```python
from build123d import *

# Parameters (mm, degrees)
F0_W      = 101.5
F0_H      = 85
F1_DEPTH  = 15.875
F3_DEPTH  = 25
F4_W      = 78.5
F4_H      = 15.875
F5_DEPTH  = 3.5
F6_W      = 78.5
F6_H      = 15.875
F7_DEPTH  = 3.5
F8_R      = 1.5
F8_W      = 66.5
F8_H      = 3
F8_W_2    = 72.5
F9_DEPTH  = 25
F10_W     = 72.5
F10_H     = 3
F10_W_2   = 66.5
F10_R     = 1.5
F11_DEPTH = 25
F12_R     = 2.5
F13_DEPTH = 5
F14_R     = 2.5
F15_DEPTH = 5
F16_R     = 2.5
F17_DEPTH = 5
F18_R     = 2.5
F19_DEPTH = 5
F20_R     = 1.5
F21_DEPTH = 10


with BuildPart() as f1:
    # F0 (on Front) → F1 (new body)
    with BuildSketch(Plane.XZ):
        Rectangle(F0_W, F0_H)
    extrude(amount=F1_DEPTH)

    # F2 (on face) → F3 (cut)
    with BuildSketch(Plane.XZ.offset(15.875)):
        with BuildLine():
            Line((-45.75, 31), (-45.75, -31))
            ThreePointArc((-45.75, -31), (-43.846194, -35.596194), (-39.25, -37.5))
            Line((-39.25, -37.5), (39.25, -37.5))
            ThreePointArc((39.25, -37.5), (43.846194, -35.596194), (45.75, -31))
            Line((45.75, -31), (45.75, 31))
            ThreePointArc((45.75, 31), (43.846194, 35.596194), (39.25, 37.5))
            Line((39.25, 37.5), (-39.25, 37.5))
            ThreePointArc((-39.25, 37.5), (-43.846194, 35.596194), (-45.75, 31))
        make_face()
    extrude(amount=-F3_DEPTH, mode=Mode.SUBTRACT)

    # F4 (on face) → F5 (cut)
    with BuildSketch(Plane.XY.offset(42.5)):
        with Locations((0, -7.9375)):
            Rectangle(F4_W, F4_H)
    extrude(amount=-F5_DEPTH, mode=Mode.SUBTRACT)

    # F6 (on face) → F7 (cut)
    with BuildSketch(Plane(origin=(0, 0, -42.5), x_dir=(1, 0, 0), z_dir=(0, 0, -1))):
        with Locations((0, 7.9375)):
            Rectangle(F6_W, F6_H)
    extrude(amount=-F7_DEPTH, mode=Mode.SUBTRACT)

    # F8 (on face) → F9 (cut)
    with BuildSketch(Plane.XY.offset(39)):
        with Locations((34.75, -4.5)):
            Circle(F8_R)
        with Locations((-3, -4.5)):
            Rectangle(F8_W, F8_H)
        with Locations((0, -10.5)):
            Rectangle(F8_W_2, F8_H)
    extrude(amount=-F9_DEPTH, mode=Mode.SUBTRACT)

    # F10 (on face) → F11 (cut)
    with BuildSketch(Plane(origin=(0, 0, -39), x_dir=(1, 0, 0), z_dir=(0, 0, -1))):
        with Locations((0, 10.5)):
            Rectangle(F10_W, F10_H)
        with Locations((3, 4.5)):
            Rectangle(F10_W_2, F10_H)
        with Locations((-34.75, 4.5)):
            Circle(F10_R)
    extrude(amount=-F11_DEPTH, mode=Mode.SUBTRACT)

    # F12 (on face) → F13 (cut)
    with BuildSketch(Plane(origin=(0, 0, -42.5), x_dir=(1, 0, 0), z_dir=(0, 0, -1))):
        with Locations((-45, 7.9375)):
            Circle(F12_R)
    extrude(amount=-F13_DEPTH, mode=Mode.SUBTRACT)

    # F14 (on face) → F15 (cut)
    with BuildSketch(Plane(origin=(0, 0, -42.5), x_dir=(1, 0, 0), z_dir=(0, 0, -1))):
        with Locations((45, 7.9375)):
            Circle(F14_R)
    extrude(amount=-F15_DEPTH, mode=Mode.SUBTRACT)

    # F16 (on face) → F17 (cut)
    with BuildSketch(Plane.XY.offset(42.5)):
        with Locations((-45, -7.9375)):
            Circle(F16_R)
    extrude(amount=-F17_DEPTH, mode=Mode.SUBTRACT)

    # F18 (on face) → F19 (cut)
    with BuildSketch(Plane.XY.offset(42.5)):
        with Locations((45, -7.9375)):
            Circle(F18_R)
    extrude(amount=-F19_DEPTH, mode=Mode.SUBTRACT)

    # F20 (on face) → F21 (cut)
    with BuildSketch(Plane.XZ.offset(15.875)):
        with Locations((-48.25, 25)):
            Circle(F20_R)
        with Locations((-48.25, 0)):
            Circle(F20_R)
        with Locations((-48.25, -25)):
            Circle(F20_R)
        with Locations((48.25, -25)):
            Circle(F20_R)
        with Locations((48.25, 0)):
            Circle(F20_R)
        with Locations((48.25, 25)):
            Circle(F20_R)
    extrude(amount=-F21_DEPTH, mode=Mode.SUBTRACT)


solid = f1.part
```
Check sheet for the modelled part. Datum: model origin and axes. Units: mm. A direction names the side the tool comes from. Round coordinates to 2 decimals unless told otherwise and drop trailing zeros. Write each loop counter-clockwise with the first axis right and the second up, starting at its lowest first coordinate (ties: lowest second). Pieces come first, ordered by that corner, then holes. Notation, with made-up numbers: (-16.75, 36.5) -> (17.25, 36.5) arc R15 ccw to (17.25, 50.5) -> close; hole circle Ø4 at (-1.75, -18.75). An arc over 180 degrees is marked (long way). One line per question, with ' | ' between items. Start each with the question number.
1. Set-up check for faces 4 (the face through (45, -8, 37.5)), 5 (the face through (39.25, -8, -41)), 6 (the face through (-43.795, -8.049, 35.646)), 7 (the face through (48, -5.875, -25)): record each of +Z, -Z, +X, -X, +Y, -Y from which the full face is reachable in a straight line by a thin tool's end or side.
2. Release check for a two-part mould opening along X. For faces 1 (the face through (-48, -8, 42.5)), 2 (the face through (47.309, -8.895, 40.035)), 3 (the face through (50.75, -8, -1)) record: +X half, -X half, draft (parallel to the pull), parting line (faces both ways), or undercut.
3. Sectioned sample at A-A, the plane x = -31.5. Record the cut outline in (y, z) (3 decimals).
4. Sectioned sample at C-C, the plane z = -25. Record the cut outline in (x, y) (3 decimals), then the cut area to 4 significant figures.
5. Depth check by flat-ended pin: pin 1 (2.5 mm diameter, centred on x = -48.25, z = 25, fed in from -Y) (3 decimals); pin 2 (1.5 mm diameter, centred on x = -16.5, y = -8.5, fed in from -Z); pin 3 (2.5 mm diameter, centred on x = -45, y = -7.5, fed in from -Z); pin 4 (8 mm diameter, centred on x = 39, z = 31, fed in from -Y). Enter the tip coordinate at first touch or a pass-through.
6. Scan lines: line 1 along Z through (x, y) = (-48.25, -12.5); line 2 along X through (y, z) = (-14.25, 4); line 3 along Z through (x, y) = (-13.5, -14.5). Record each from-to range of solid material in increasing order. Write a range as from..to.
7. Sectioned sample at B-B, the plane y = -14.75. Record the cut outline in (x, z).
8. Sectioned sample at D-D, the plane z = 17. Record the cut outline in (x, y) (3 decimals), then the cut area to 3 significant figures.
Taken from the geometry:
1) face 4: +Z | face 5: -Z, +Y, -Y | face 6: +Y, -Y | face 7: -Y
2) face 1: draft | face 2: undercut | face 3: +X half
3) outline: (-15.875, -39) -> (-12, -39) -> (-12, -37.5) -> (-15.875, -37.5) -> close; (-15.875, 37.5) -> (-12, 37.5) -> (-12, 39) -> (-15.875, 39) -> close; (-9, -39) -> (0, -39) -> (0, -37.5) -> (-9, -37.5) -> close; (-9, 37.5) -> (-6, 37.5) -> (-6, 39) -> (-9, 39) -> close; (-3, 37.5) -> (0, 37.5) -> (0, 39) -> (-3, 39) -> close
4) outline: (-50.75, -15.875) -> (-49.75, -15.875) -> (-49.75, -5.875) -> (-46.75, -5.875) -> (-46.75, -15.875) -> (-45.75, -15.875) -> (-45.75, 0) -> (-50.75, 0) -> close; (45.75, -15.875) -> (46.75, -15.875) -> (46.75, -5.875) -> (49.75, -5.875) -> (49.75, -15.875) -> (50.75, -15.875) -> (50.75, 0) -> (45.75, 0) -> close | area: 98.75 mm^2
5) pin 1: stops at y = -5.875 | pin 2: stops at z = -39 | pin 3: stops at z = -37.5 | pin 4: passes through
6) line 1: z = -42.5..-26.5, -23.5..-1.5, 1.5..23.5, 26.5..42.5 | line 2: x = -50.75..-45.75, 45.75..50.75 | line 3: z = -39..-37.5, 37.5..39
7) outline: (-50.75, -42.5) -> (-39.25, -42.5) -> (-39.25, -39) -> (39.25, -39) -> (39.25, -42.5) -> (50.75, -42.5) -> (50.75, 42.5) -> (39.25, 42.5) -> (39.25, 39) -> (-39.25, 39) -> (-39.25, 42.5) -> (-50.75, 42.5) -> close; hole circle Ø3 at (-48.25, -25); hole circle Ø3 at (-48.25, 0); hole circle Ø3 at (-48.25, 25); hole (-45.75, -31) arc R6.5 ccw to (-39.25, -37.5) -> (39.25, -37.5) arc R6.5 ccw to (45.75, -31) -> (45.75, 31) arc R6.5 ccw to (39.25, 37.5) -> (-39.25, 37.5) arc R6.5 ccw to (-45.75, 31) -> close; hole circle Ø3 at (48.25, -25); hole circle Ø3 at (48.25, 0); hole circle Ø3 at (48.25, 25)
8) outline: (-50.75, -15.875) -> (-45.75, -15.875) -> (-45.75, 0) -> (-50.75, 0) -> close; (45.75, -15.875) -> (50.75, -15.875) -> (50.75, 0) -> (45.75, 0) -> close | area: 159 mm^2
